Design review of the part built by this model. Coordinates are the model's own, in mm. Give positions to 0.01 mm unless a question says otherwise; leave off trailing zeros. Order: outer loops, then holes, each group sorted by start corner. A loop starts at its lowest first (then second) coordinate and runs counter-clockwise, first axis right, second up. Notation, with made-up numbers: (25, 61.5) -> (57, 61.5) arc R22 cw to (57, 85.5) -> close; hole circle Ø6 at (0, 14). An arc over 180 degrees is marked (long way). One line per item, written item: value.
from build123d import *

# Parameters (mm, degrees)
SKETCH1_R           = 8.25
BOSS_EXTRUDE1_DEPTH = 5.2
SKETCH1_4_R         = 7.994032283
BOSS_EXTRUDE3_DEPTH = 6
FILLET1_R           = 10


with BuildPart() as part:
    # Sketch1 → Boss-Extrude1 (new body)
    with BuildSketch(Plane.XY):
        Circle(SKETCH1_R)
    extrude(amount=BOSS_EXTRUDE1_DEPTH)

    # Sketch1<4> → Boss-Extrude3 (add)
    with BuildSketch(Plane.XY):
        Circle(SKETCH1_4_R)
    extrude(amount=BOSS_EXTRUDE3_DEPTH)

    # Fillet1
    # the kernel refuses this fillet: 10 mm, written as the material it takes off along each edge
    with BuildSketch(Plane(origin=(0, 0, 6), x_dir=(1, 0, 0), z_dir=(0, -1, 0))) as fillet1_piece_1:
        with BuildLine():
            CenterArc((4.074848695, -10), FILLET1_R, 66.926081934, 23.073918066)
            Line((4.074848695, 0), (4.074848695, 0.2))
            Line((4.074848695, 0.2), (7.994032283, 0.2))
            Line((7.994032283, 0.2), (8.194032283, 0))
            ThreePointArc((8.194032283, 0), (8.194032283, -0.4), (8.072415955, -0.616))
            Line((8.072415955, -0.616), (7.994032283, -0.8))
        make_face()
    revolve(axis=Axis((0, 0, 6), (0, 0, 1)), mode=Mode.SUBTRACT)


solid = part.part
Item 1: Add section A-A on z = 2.75. Give the boundary of the cut face in (x, y), plus the area to 3 significant figures.
Returned:
outline: circle Ø16.5 at (0, 0)
area: 214 mm²
Item 2: Clearance check with flat-ended pins moving along their axes: P1, Ø3, axis at y = -5.5, z = 4.5, coming from the -X side; P2, Ø2, axis at y = 5.5, z = 4, coming from the -X side; P3, Ø1.5, axis at x = -2, z = 1, coming from the -Y side. State where each tip first meets the part, or that it passes through.
Returned:
P1: x = -7.22
P2: x = -6.91
P3: y = -8.15
Item 3: To check wall thickness, follow line 1 along Y through (x, z) = (0.5, 5); line 2 along Y through (x, z) = (3, 2.5); line 3 along Z through (x, y) = (-3.25, 5.5). State the ranges of each line that lie inside material, in increasing order. Write a range as from..to.
Returned:
line 1: -8.23..8.23
line 2: -7.69..7.69
line 3: 0..5.73
